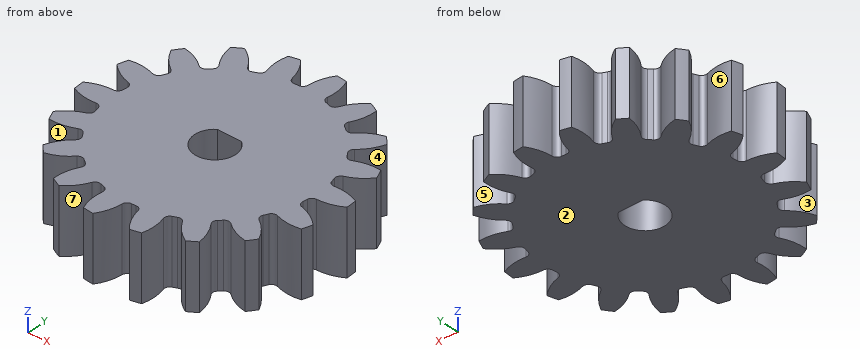
from build123d import *

# Parameters (mm, degrees)
SKETCH3_R         = 12.7
GEARBODY_DEPTH    = 6.35
TOOTHCUT_DEPTH    = 7.35
CIRPATTERN1_COUNT = 18
BORE_DEPTH        = 12.7


with BuildPart() as part:
    # Sketch3 → gearBody (new body)
    with BuildSketch(Plane.XY):
        Circle(SKETCH3_R)
    extrude(amount=GEARBODY_DEPTH)

    # Sketch2 → toothCut (cut, through all)
    with BuildSketch(Plane.XY):
        with BuildLine():
            ThreePointArc((9.781229257, -1.205205904), (9.806057787, -0.982953571), (9.825836884, -0.760195085))
            ThreePointArc((9.825836884, -0.760195085), (9.980803767, -0.435792976), (10.31355819, -0.299682883))
            ThreePointArc((10.31355819, -0.299682883), (12.38209996, 0.246018063), (13.970369973, 1.679214819))
            ThreePointArc((13.970369973, 1.679214819), (14.000763839, -1.403428484), (13.359117821, -4.418706897))
            ThreePointArc((13.359117821, -4.418706897), (12.0869153, -2.698778026), (10.167842346, -1.753360882))
            ThreePointArc((10.167842346, -1.753360882), (9.868724138, -1.553912241), (9.781229257, -1.205205904))
        make_face()
    toothcut = extrude(amount=TOOTHCUT_DEPTH, mode=Mode.SUBTRACT)

    # CirPattern1: toothCut ×18 about axis
    cirpattern1_axis = Axis((0, 0, 0), (0, 0, 1))
    for i in range(1, CIRPATTERN1_COUNT):
        add(toothcut.rotate(cirpattern1_axis, i * 360 / CIRPATTERN1_COUNT), mode=Mode.SUBTRACT)

    # boreDia → bore (cut, symmetric)
    with BuildSketch(Plane.XY):
        with BuildLine():
            Line((-1.2, 1.60000008), (1.2, 1.60000008))
            ThreePointArc((1.2, 1.60000008), (0, -2.000000064), (-1.2, 1.60000008))
        make_face()
    extrude(amount=BORE_DEPTH, both=True, mode=Mode.SUBTRACT)


solid = part.part
Here's how the part is built. I have some questions about the finished solid (model axes, mm). Face numbers are marked on the shaded views. A direction names the side the tool comes from. Coordinates: 2 decimals unless noted, no trailing zeros. Write each loop counter-clockwise with the first axis right and the second up, starting at its lowest first coordinate (ties: lowest second). Pieces come first, ordered by that corner, then holes. Notation, with made-up numbers: (-32, -14.75) - (-14, -14.75) arc R29 cw to (-14, 8.25) - close; hole circle Ø1 at (81, 3.25). An arc over 180 degrees is marked (long way). Use one line per item in the form item = value.
1) Suppose I cut it at A-A, the plane y = 0. Write out the boundary of the cut face in (x, z).
Solved:
outline = (-11.85, 0) - (-2, 0) - (-2, 6.35) - (-11.85, 6.35) - close; (2, 0) - (11.85, 0) - (11.85, 6.35) - (2, 6.35) - close
2) On a 3-axis mill with a long thin cutter (end or side, diameter ignored), from which of +Z, -Z, +X, -X, +Y, -Y can I reach the whole of each face in a straight line? I mean the marked faces 4, 5, 6 and 7. Say none if no direction works.
Solved:
face_4 = +Z, -Z, +X
face_5 = +Z, -Z, +Y
face_6 = +Z, -Z
face_7 = +Z, -Z, -Y
3) I need wall thicknesses on line 1 (X direction, y = 10.5, z = 1.5); line 2 (X direction, y = -10.25, z = 4.25); line 3 (Y direction, x = -9, z = 4.5). Which ranges of each line are inside material? Lowest first, please.
Solved:
line_1 = -7.14 to -6.25, -3.74 to -1.56, -0.03 to 2.13, 3.92 to 5.96
line_2 = -5.92 to -3.76, -2.11 to 0.05, 1.5 to 3.7, 5.91 to 7.5
line_3 = -8.96 to -7.48, -5.24 to 4.02, 5.15 to 7.59
4) I'm going to push flat-ended pins straight in: P1, Ø1, axis at y = -2.5, z = 1, coming from the -X side; P2, Ø1, axis at y = 10, z = 3, coming from the -X side; P3, Ø2, axis at y = 3.5, z = 5, coming from the -X side. Where does each tip first touch, or does it pass through?
Solved:
P1 = -9.71
P2 = -7.57
P3 = -12.35
5) Thinking about a two-plate mould opening in X: for the marked faces 1, 2 and 3, which applies, released by +X, released by -X, zero draft, split by the parting line, or undercut?
Solved:
face_1 = undercut
face_2 = zero draft
face_3 = released by -X
